Autodesk Inventor part; units mm, degrees
ref_plane "Work Plane1" through (0, -12.25, 0) normal (0, 1, 0) x (-1, 0, 0)
ref_plane "Work Plane2" through (0, -12.25, 0) normal (0, 1, 0) x (-1, 0, 0)
ref_plane "YZ Plane" through (0, 0, 0) normal (1, 0, 0) x (0, 1, 0)
sketch "Sketch1" plane through (0, 0, 0) normal (0, 0, 1) x (1, 0, 0)
  circle A0 centre (0, 0) radius 12.25
  circle A1 centre (0, 0) radius 11.5
  dimension "d0" = 24.5
  dimension "d1" = 23
extrude "Extrusion1" add sketch "Sketch1" along normal blind 49.5
sketch "Sketch2" plane through (0, 0, 49.5) normal (0, 0, 1) x (1, 0, 0)
  line L0 (-17.15, 0) -> (17.15, 0)
  line L1 (0, -17.15) -> (0, 17.15)
  line L2 (0, 0) -> (-11.8326, 3.1705)
  line L3 (0, 0) -> (-8.6621, -8.6621)
  line L4 (0, 0) -> (11.8326, 3.1705)
  line L5 (0, 0) -> (8.6621, -8.6621)
  arc A0 (11.8326, 3.1705) -> (-11.8326, 3.1705) centre (0, 0) ccw
  arc A1 (-8.6621, -8.6621) -> (8.6621, -8.6621) centre (0, 0) ccw
  dimension "d4" = 15
  dimension "d5" = 45
extrude "Extrusion2" cut sketch "Sketch2" against normal blind 10
sketch "Sketch3" plane through (0, 0, 0) normal (0, 0, -1) x (-1, 0, 0)
  circle A0 centre (0, 0) radius 12.25
extrude "Extrusion3" add sketch "Sketch3" along normal blind 1
sketch "Sketch4" plane through (0, 0, -1) normal (0, 0, -1) x (-1, 0, 0)
  circle A0 centre (0, 0) radius 12.25
hole "Hole1" at (0, 0, -1) direction (0, 0, 1) diameter 10 end through all
ref_plane "Work Plane1" through (0, -12.25, 0) normal (0, 1, 0) x (-1, 0, 0)
sketch "Sketch5" plane through (0, -12.25, 0) normal (0, 1, 0) x (-1, 0, 0)
  line L0 (12.25, -1) -> (-12.25, -1)
  line L1 (11.5, 0) -> (-11.5, 0)
  line L2 (-5, 0) -> (-5, -1)
  line L3 (5, 0) -> (5, -1)
  line L4 (12.25, -1) -> (12.25, 49.5)
  line L5 (-12.25, -1) -> (-12.25, 49.5)
  line L6 (12.25, -1) -> (-12.25, -1)
  line L7 (11.8326, 49.5) -> (11.8326, 39.5)
  line L8 (11.8326, 39.5) -> (-11.8326, 39.5)
  line L9 (-11.8326, 39.5) -> (-11.8326, 49.5)
  line L10 (-11.8326, 49.5) -> (-8.6621, 49.5)
  line L11 (-8.6621, 49.5) -> (-8.6621, 39.5)
  line L12 (-8.6621, 39.5) -> (8.6621, 39.5)
  line L13 (8.6621, 39.5) -> (8.6621, 49.5)
  line L14 (8.6621, 49.5) -> (11.8326, 49.5)
  line L15 (11.5, 0) -> (11.5, 49.5)
  line L16 (0, -13.4846) -> (0, 73.9076)
  line L17 (7.5, 49) -> (-7.5, 49)
  line L18 (-7.5, 49) -> (-7.5, -1)
  line L19 (-7.5, -1) -> (7.5, -1)
  line L20 (7.5, -1) -> (7.5, 49)
  point P0 (0, 0)
  point P1 (0, 49)
  point P2 (0, 0)
  dimension "d17" = 15
  dimension "d18" = 50
extrude "Extrusion4" [suppressed]
ref_plane "Work Plane2" through (0, -12.25, 0) normal (0, 1, 0) x (-1, 0, 0)
sketch "Sketch8" plane through (0, 0, -1) normal (0, 0, -1) x (-1, 0, 0)
  circle A0 centre (0, 0) radius 5
  circle A1 centre (0, 0) radius 7.5
  dimension "d26" = 15
extrude "Extrusion7" add sketch "Sketch8" along normal blind 13.923
sketch "Sketch7" plane through (0, 0, 49.5) normal (0, 0, 1) x (1, 0, 0)
  arc A0 (8.6621, -8.6621) -> (11.8326, 3.1705) centre (0, 0) ccw
  arc A1 (8.1317, -8.1317) -> (11.1081, 2.9764) centre (0, 0) ccw
  line L0 (8.1317, -8.1317) -> (8.6621, -8.6621)
  line L1 (-10.4211, -8.1317) -> (11.1081, -8.1317)
  line L2 (11.1081, -8.1317) -> (11.1081, -13.0652)
  line L3 (11.1081, -13.0652) -> (-10.4211, -13.0652)
  line L4 (-10.4211, -13.0652) -> (-10.4211, -8.1317)
extrude "Extrusion6" cut sketch "Sketch7" against normal through all
properties part number "ss_inner_guide"
Geometry: final body of the model. Coordinates: model frame, mm. Give positions to 0.01 mm unless a question says otherwise; leave off trailing zeros. Loops run counter-clockwise (first coordinate to the right, second up) from the corner with the lowest first, then second, coordinate; pieces in that order, holes last. Notation, with made-up numbers: (71, 40) -> (100, 40) arc R21 cw to (100, 79) -> close; hole circle Ø9 at (85.25, -2). An arc over 180 degrees is marked (long way). Return JSON: item names as keys, results as strings.
Item 1: Section A-A, the plane x = 0. Output: boundary loops of the cut face in (y, z).
Filled in:
{"outline": "(-8.13, -1) -> (-7.5, -1) -> (-7.5, -14.92) -> (-5, -14.92) -> (-5, 0) -> (-8.13, 0) -> close; (5, -14.92) -> (7.5, -14.92) -> (7.5, -1) -> (12.25, -1) -> (12.25, 39.5) -> (11.5, 39.5) -> (11.5, 0) -> (5, 0) -> close"}
Item 2: Mould query, pull axis Y, two halves, no side actions, for faces 1 (the cylindrical face through (-0.379, 11.494, 24.404)), 2 (the cylindrical face through (7.493, -0.33, -7.864)), 3 (the flat face through (-11.3, -2.9, 49.5)), 4 (the flat face through (0, 6, 0)). Classes: released by +Y, released by -Y, zero draft, split by the parting line, or undercut.
Filled in:
{"face 1": "undercut", "face 2": "split by the parting line", "face 3": "zero draft", "face 4": "undercut"}
Item 3: Section B-B, the plane y = 0. Output: boundary loops of the cut face in (x, z), plus the area to 3 significant figures.
Filled in:
{"outline": "(-12.25, -1) -> (-7.5, -1) -> (-7.5, -14.92) -> (-5, -14.92) -> (-5, 0) -> (-11.5, 0) -> (-11.5, 49.5) -> (-12.25, 49.5) -> close; (5, -14.92) -> (7.5, -14.92) -> (7.5, -1) -> (12.25, -1) -> (12.25, 49.5) -> (11.5, 49.5) -> (11.5, 0) -> (5, 0) -> close", "area": "158 mm^2"}
Item 4: Section C-C, the plane z = -7.5. Output: boundary loops of the cut face in (x, y).
Filled in:
{"outline": "circle Ø15 at (0, 0); hole circle Ø10 at (0, 0)"}
Item 5: Line query: line 1 (X direction, y = 0.25, z = -11); line 2 (X direction, y = 0.5, z = 42.5); line 3 (Y direction, x = 0, z = -6). Output: solid intervals per line, ascending.
Filled in:
{"line 1": "-7.5 to -4.99, 4.99 to 7.5", "line 2": "-12.24 to -11.49, 11.49 to 12.24", "line 3": "-7.5 to -5, 5 to 7.5"}
Item 6: Pin query (flat end, axial travel): P1, Ø10, axis at x = 9, z = 38.5, coming from the +Y side; P2, Ø1.5, axis at y = -5.5, z = 16.5, coming from the +X side; P3, Ø6, axis at x = 3, y = 1.5, coming from the +Z side. Return the tip coordinate at first contact, or that it passes through.
Filled in:
{"P1": "y = 11.58", "P2": "x = 11.29", "P3": "z = 0"}
Item 7: Section D-D, the plane y = 10.75. Output: boundary loops of the cut face in (x, z), plus the area to 3 significant figures.
Filled in:
{"outline": "(-5.87, -1) -> (5.87, -1) -> (5.87, 39.5) -> (4.09, 39.5) -> (4.09, 0) -> (-4.09, 0) -> (-4.09, 39.5) -> (-5.87, 39.5) -> close", "area": "153 mm^2"}
